Could you check a few things on this drawing? It's one solid part, dimensions in mm from its lowest x, y, z. Give positions to 0.01 mm unless a question says otherwise; leave off trailing zeros. Order: outer loops, then holes, each group sorted by start corner. A loop starts at its lowest first (then second) coordinate and runs counter-clockwise, first axis right, second up. Notation, with made-up numbers: M 14,-39 L 32,-39 A15 ccw 32,-25 Z; hole C 67.25,71 d5. An arc over 180 degrees is marked long. Use CSV: the item, a comma, the result in double quotes. Start each with the question number.
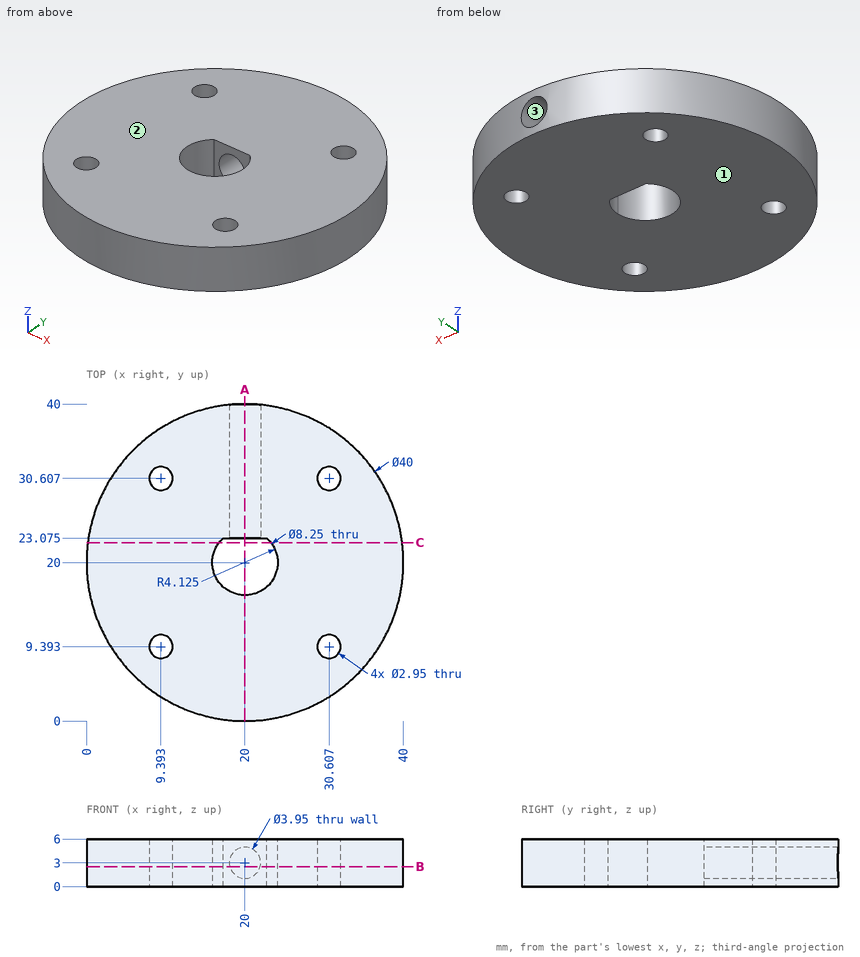
Q1. Imagine slicing it at A-A, the plane x = 20. Please give me the cut outline in (y, z) (1 decimal).
Q2. Imagine slicing it at C-C, the plane y = 22.5. Please give me the cut outline in (x, z).
Q3. Imagine slicing it at B-B, the plane z = 2.5. Count the separate pieces of the cut face and the enclosed holes in it, then the cut area to 3 significant figures.
Q4. For P1, Ø1.8, axis at x = 9.39, y = 9.39, coming from the +Z side; P2, Ø3.5, axis at x = 30.61, y = 9.39, coming from the +Z side; P3, Ø2, axis at y = 8.5, z = 1, coming from the +X side; P4, Ø1.5, axis at x = 21.5, z = 3, coming from the -Y side, each with a flat end and sliding along its axis, tell me the tip position at first contact or that it passes through.
Q5. We'd pull the mould along Z, two halves only. Please class the marked faces 1, 2 and 3: pulls with the +Z half, pulls with the -Z half, needs draft (parallel to the pull), parting line crosses it, or undercut.
Q6. I need wall thicknesses on line 1 (Y direction, x = 8.5, z = 2.5) (1 decimal); line 2 (X direction, y = 10, z = 5.75). Which ranges of each line are inside material? Lowest first, please. Write a range as [from, to].
Reply:
1,outline,"M 0,0 L 15.9,0 L 15.9,6 L 0,6 Z; M 23.1,0 L 40,0 L 40,1 L 23.1,1 Z; M 23.1,5 L 40,5 L 40,6 L 23.1,6 Z"
2,outline,"M 0.16,0 L 16.72,0 L 16.72,6 L 0.16,6 Z; M 23.28,0 L 39.84,0 L 39.84,6 L 23.28,6 Z"
3,separate pieces,"1"
3,enclosed holes,"4"
3,area,"1,120 mm^2"
4,P1,"passes through"
4,P2,"stops at z = 6"
4,P3,"stops at x = 37.02"
4,P4,"stops at y = 0.01"
5,face 1,"pulls with the -Z half"
5,face 2,"pulls with the +Z half"
5,face 3,"undercut"
6,line 1,"y = [3.6, 8.2], [10.6, 29.4], [31.8, 36.4]"
6,line 2,"x = [2.68, 8.05], [10.74, 29.26], [31.95, 37.32]"
